Read the model definition and answer for the solid it produces. Units are mm, in the model's axes. A direction names the side the tool comes from. Coordinates: 2 decimals unless noted, no trailing zeros. Loops run counter-clockwise (first coordinate to the right, second up) from the corner with the lowest first, then second, coordinate; pieces in that order, holes last. Notation, with made-up numbers: (-6.75, 89) - (51.25, 89) arc R25 ccw to (51.25, 125) - close; hole circle Ø3 at (63, 60). An arc over 180 degrees is marked (long way). Use CSV: the item, a comma, the result in double quotes.
```python
from build123d import *

# Parameters (mm, degrees)
PAD002_DEPTH = 10
SKETCH001_W  = 8.2
SKETCH001_H  = 19.7
PAD001_DEPTH = 11.6
PAD_DEPTH    = 12.5
PAD003_DEPTH = 2.5


with BuildPart() as escuadra:
    # Sketch002 → Pad002 (new body)
    with BuildSketch(Plane.YZ.offset(22.85)):
        Polygon((-44, 12.5), (-11.6, 12.5), (-11.6, 52.5), align=None)
    extrude(amount=PAD002_DEPTH)


with BuildPart() as obj1:
    # Sketch001 → Pad001 (new body)
    with BuildSketch(Plane.XZ):
        Polygon((0, 0), (0, 52.4), (12.3, 52.4), (12.3, 65.7), (38.7, 65.7), (38.7, 51.9), (51.4, 51.9), (51.4, 0), align=None)
        with Locations((10.7, 36.25)):
            Rectangle(SKETCH001_W, SKETCH001_H, mode=Mode.SUBTRACT)
    extrude(amount=PAD001_DEPTH)


with BuildPart() as escuadra_central:
    # Sketch → Pad (new body)
    with BuildSketch(Plane.XY):
        with BuildLine():
            Line((0, 0), (51.3, 0))
            Line((51.3, 0), (51.3, -31.6))
            Line((51.3, -31.6), (47.8, -31.6))
            Line((47.8, -31.6), (46, -44.070766))
            Line((46, -44.070766), (15.5, -44.070766))
            ThreePointArc((7.5, -36.070766), (9.843146, -41.72762), (15.5, -44.070766))
            Line((7.5, -36.070766), (7.5, -32.5))
            Line((7.5, -32.5), (0, -32.5))
            Line((0, -32.5), (0, 0))
        make_face()
    extrude(amount=PAD_DEPTH)

    # Sketch003 → Pad003 (new body)
    with BuildSketch(Plane.XY.offset(12.5)):
        with BuildLine():
            Line((4.5, -11.6), (16.1, -11.6))
            Line((16.1, -11.6), (14.3, -23.6))
            ThreePointArc((6.3, -23.6), (10.3, -27.6), (14.3, -23.6))
            Line((6.3, -23.6), (4.5, -11.6))
        make_face()
    extrude(amount=PAD003_DEPTH)

    # Fusion: union escuadra, obj1
    add(escuadra.part)
    add(obj1.part)


solid = escuadra_central.part
```
Q1. The part is cut by section D-D on x = 42.5. Determine the outline of the cut face in (y, z), and give its area (3 significant figures).
Reported:
outline,"(-44.07, 0) - (0, 0) - (0, 51.9) - (-11.6, 51.9) - (-11.6, 12.5) - (-44.07, 12.5) - close"
area,"1,010 mm²"
Q2. A tool of negligible diameter and unlimited length cuts with its end or side. For faces 4 (the face through (32.85, -21, 24)), 5 (the face through (20, -28, 12.5)), 6 (the face through (4, -32.5, 6)), from which of +Z, -Z, +X, -X, +Y, -Y can it reach the whole face along a straight path? Write none if from no direction.
Reported:
face 4,"+Z, +X, -Y"
face 5,"+Z, -Y"
face 6,"+Z, -Z, -X, -Y"
Q3. For a pull along X with two mould halves and no side action, classify faces 1 (the face through (11, -6, 46.1)), 2 (the face through (45, -6, 51.9)), 3 (the face through (38.7, -6, 59)) as +X half, -X half, draft (parallel to the pull), parting line (faces both ways), or undercut.
Reported:
face 1,"undercut"
face 2,"draft"
face 3,"+X half"
Q4. The part is cut by section B-B on z = 34.5. Determine the outline of the cut face in (x, y), and give its area (3 significant figures).
Reported:
outline,"(0, -11.6) - (6.6, -11.6) - (6.6, 0) - (0, 0) - close; (14.8, -11.6) - (22.85, -11.6) - (22.85, -26.18) - (32.85, -26.18) - (32.85, -11.6) - (51.4, -11.6) - (51.4, 0) - (14.8, 0) - close"
area,"647 mm²"
Q5. Find the intervals of material crossed by probe 1 along Z at (x, y) = (10, -13.5); probe 2 along X at (y, z) = (-22, 35); probe 3 along Z at (x, y) = (18, -36.5), in increasing order. Write a range as [from, to].
Reported:
probe 1,"z = [0, 15]"
probe 2,"x = [22.85, 32.85]"
probe 3,"z = [0, 12.5]"
Q6. Given P1, Ø1.8, axis at x = 49.5, z = 3, coming from the -Y side; P2, Ø3, axis at x = 34.5, y = -34, coming from the +Z side; P3, Ø13, axis at x = 9.5, y = -23, coming from the +Z side, each flat-ended and moving along its own axis, determine where each tip first touches the part or whether it passes through.
Reported:
P1,"stops at y = -31.6"
P2,"stops at z = 12.5"
P3,"stops at z = 15"
Q7. The part is cut by section A-A on y = -8. Determine the outline of the cut face in (x, z), and give its area (3 significant figures).
Reported:
outline,"(0, 0) - (51.4, 0) - (51.4, 51.9) - (38.7, 51.9) - (38.7, 65.7) - (12.3, 65.7) - (12.3, 52.4) - (0, 52.4) - close; hole (6.6, 26.4) - (14.8, 26.4) - (14.8, 46.1) - (6.6, 46.1) - close"
area,"2,880 mm²"
Q8. The part is cut by section C-C on z = 19.5. Determine the outline of the cut face in (x, y).
Reported:
outline,"(0, -11.6) - (22.85, -11.6) - (22.85, -38.33) - (32.85, -38.33) - (32.85, -11.6) - (51.4, -11.6) - (51.4, 0) - (0, 0) - close"
